Read the model definition and answer for the solid it produces. Units are mm, in the model's axes. A direction names the side the tool comes from. Coordinates: 2 decimals unless noted, no trailing zeros. Loops run counter-clockwise (first coordinate to the right, second up) from the corner with the lowest first, then second, coordinate; pieces in that order, holes last. Notation, with made-up numbers: (-28.5, 26) -> (-3.5, 26) arc R19 ccw to (-3.5, 36) -> close; hole circle Ø3 at (-5.75, -10). An arc over 180 degrees is marked (long way). Answer as a JSON object with one key per item and string values. Group by question number.
Q1. Straight lines are drawn through the part: line 1 along Y through (x, z) = (17.5, 9); line 2 along X through (y, z) = (0.95, 6); line 3 along X through (y, z) = (23.25, -16). For each, find the intervals that lie inside material, in ascending order. Write a range as [from, to].
Q2. Determine the mould class of faces 3 (the cylindrical face through (-10.81, 8.583, -15.364)), 4 (the flat face through (30, 2, -5)), 5 (the flat face through (-6.3, 7.7, 11.5)) for opening direction X: released by +X, released by -X, zero draft, split by the parting line, or undercut.
Q3. The part is cut by section A-A on z = -4.5. Write down the section's boundary in (x, y).
Q4. The part is cut by section B-B on x = -28.5. Write down the section's boundary in (y, z).
Q5. For faces 1 (the flat face through (-6.3, 7.7, -21.5)), 2 (the flat face through (15, 4, -5)), determine the directions among +Z, -Z, +X, -X, +Y, -Y from which every point of the face is accessible in a straight line to the end or side of a thin tool.
Q6. Each of these flat-tipped pins is pushed along its axis until it touches: P1, Ø5, axis at x = 23.32, z = 6, coming from the +Y side; P2, Ø3, axis at y = 25, z = -3.5, coming from the -X side; P3, Ø12, axis at y = 10, z = 3, coming from the -X side. Where does it stop, or does it pass through?
from build123d import *

# Parameters (mm, degrees)
SKETCH1_W           = 50
SKETCH1_H           = 23
BOSS_EXTRUDE1_DEPTH = 20
CUT_EXTRUDE3_DEPTH  = 30
CUT_EXTRUDE4_DEPTH  = 30
SKETCH9_W           = 23
SKETCH9_H           = 4
BOSS_EXTRUDE2_DEPTH = 20
BOSS_EXTRUDE3_DEPTH = 10
SKETCH14_R          = 1.65
CUT_EXTRUDE6_DEPTH  = 10
SKETCH22_W          = 33
SKETCH22_H          = 4
BOSS_EXTRUDE4_DEPTH = 5
CUT_EXTRUDE7_DEPTH  = 5


with BuildPart() as part:
    # Sketch1 → Boss-Extrude1 (new body)
    with BuildSketch(Plane(origin=(0, 0, 0), x_dir=(1, 0, 0), z_dir=(0, 1, 0))):
        Rectangle(SKETCH1_W, SKETCH1_H)
    extrude(amount=BOSS_EXTRUDE1_DEPTH)

    # Sketch2 → Cut-Extrude3 (cut)
    with BuildSketch(Plane.XY.offset(11.5)):
        Polygon((0, 0), (-25, 14.43375673), (-25, 0), align=None)
        Polygon((1.07179677, 4), (25, 4), (25, 20), (-25, 20), (-25, 19.052558883), align=None)
    extrude(amount=-CUT_EXTRUDE3_DEPTH, mode=Mode.SUBTRACT)

    # Sketch4 → Cut-Extrude4 (cut)
    with BuildSketch(Plane.XY.offset(11.5)):
        Polygon((-25, 14.43375673), (-23, 17.897858345), (-25, 19.052558883), align=None)
    extrude(amount=-CUT_EXTRUDE4_DEPTH, mode=Mode.SUBTRACT)

    # Sketch9 → Boss-Extrude2 (add)
    with BuildSketch(Plane(origin=(-25, 14.43375673, 0), x_dir=(0, 0, 1), z_dir=(-0.8660254037844407, 0.4999999999999965, 0))):
        with Locations((0, 2)):
            Rectangle(SKETCH9_W, SKETCH9_H)
    extrude(amount=BOSS_EXTRUDE2_DEPTH)

    # Sketch11 → Boss-Extrude3 (add)
    with BuildSketch(Plane(origin=(0, 0, -11.5), x_dir=(-1, 0, 0), z_dir=(0, 0, -1))):
        Polygon((-25, 4), (-1.07179677, 4), (40.320508076, 27.897858345), (42.320508076, 24.43375673), (0, 0), (-25, 0), align=None)
    extrude(amount=BOSS_EXTRUDE3_DEPTH)

    # Sketch14 → Cut-Extrude6 (cut)
    with BuildSketch(Plane(origin=(2, 3.464101615, 0), x_dir=(0.866025403784438, -0.5000000000000012, 0), z_dir=(0.5000000000000011, 0.8660254037844379, 0))):
        with Locations(Location((-43.867513459, 17, 0), (0, 0, 180))):
            Circle(SKETCH14_R)
        with Locations(Location((-43.867513459, -7, 0), (0, 0, 180))):
            Circle(SKETCH14_R)
        with Locations(Location((-13.867513459, 17, 0), (0, 0, 180))):
            Circle(SKETCH14_R)
        with Locations(Location((-13.867513459, -7, 0), (0, 0, 180))):
            Circle(SKETCH14_R)
    extrude(amount=-CUT_EXTRUDE6_DEPTH, mode=Mode.SUBTRACT)

    # Sketch22 → Boss-Extrude4 (add)
    with BuildSketch(Plane(origin=(25, 0, 0), x_dir=(0, 0, -1), z_dir=(1, 0, 0))):
        with Locations((5, 2)):
            Rectangle(SKETCH22_W, SKETCH22_H)
    extrude(amount=BOSS_EXTRUDE4_DEPTH)

    # Sketch23 → Cut-Extrude7 (cut)
    with BuildSketch(Plane.XZ):
        with BuildLine():
            ThreePointArc((23.322235494, 7.62), (22.176722509, 4.854487014), (24.942235494, 6))
            Line((24.942235494, 6), (23.322235494, 6))
            Line((23.322235494, 6), (23.322235494, 7.62))
        make_face()
        with BuildLine():
            Line((23.322235494, 6), (24.942235494, 6))
            ThreePointArc((24.942235494, 6), (24.46774848, 7.145512986), (23.322235494, 7.62))
            Line((23.322235494, 7.62), (23.322235494, 6))
        make_face()
        with BuildLine():
            ThreePointArc((6.702235494, -16), (7.176722509, -17.145512986), (8.322235494, -17.62))
            Line((8.322235494, -17.62), (8.322235494, -16))
            Line((8.322235494, -16), (6.702235494, -16))
        make_face()
        with BuildLine():
            Line((8.322235494, -16), (8.322235494, -17.62))
            ThreePointArc((8.322235494, -17.62), (9.46774848, -17.145512986), (9.942235494, -16))
            ThreePointArc((9.942235494, -16), (8.322235494, -14.38), (6.702235494, -16))
            Line((6.702235494, -16), (8.322235494, -16))
        make_face()
    extrude(amount=-CUT_EXTRUDE7_DEPTH, mode=Mode.SUBTRACT)


solid = part.part
Final values:
{
 "1": {"line 1": "y = [0, 4]", "line 2": "x = [-1.65, 21.7], [24.94, 30]", "line 3": "x = [-40.27, -38.75], [-35.71, -32.27]"},
 "2": {"face 3": "undercut", "face 4": "released by +X", "face 5": "zero draft"},
 "3": {"outline": "(-42.32, 24.43) -> (0, 0) -> (30, 0) -> (30, 4) -> (1.07, 4) -> (-40.32, 27.9) -> close"},
 "4": {"outline": "(16.45, -21.5) -> (21.07, -21.5) -> (21.07, 11.5) -> (16.45, 11.5) -> close"},
 "5": {"face 1": "-Z, +X, -X, +Y, -Y", "face 2": "+Z, -Z, +X, +Y"},
 "6": {"P1": "stops at y = 4", "P2": "stops at x = -42.32", "P3": "stops at x = -27.71"}
}
